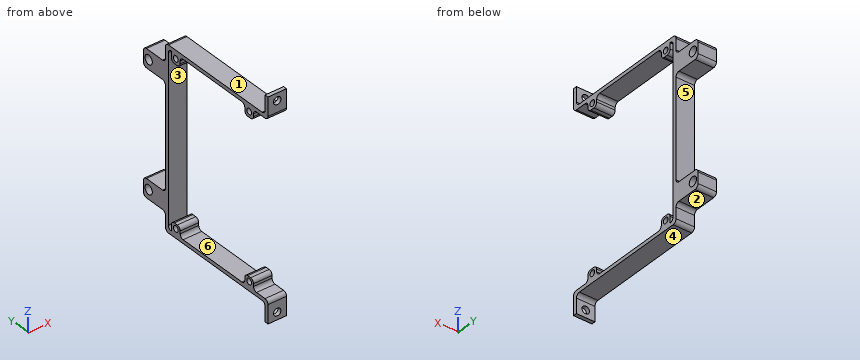
```python
from build123d import *

# Parameters (mm, degrees)
SKETCH1_W             = 10
SKETCH1_H             = 15
SKETCH1_R             = 2.5
BOSS_EXTRUDE1_DEPTH   = 10
FILLET1_R             = 2
F_4_0MM_DOWEL_HOLE1_D = 4
SKETCH4_W             = 5.416503596
SKETCH4_H             = 6
SKETCH4_R             = 1.6
BOSS_EXTRUDE2_DEPTH   = 10
FILLET1_OF_MIRROR1_R  = 2
SKETCH5_W             = 5.416503596
SKETCH5_H             = 6
SKETCH5_R             = 1.6
BOSS_EXTRUDE3_DEPTH   = 10
FILLET2_R             = 2


with BuildPart() as part:
    # Sketch1 → Boss-Extrude1 (new body)
    # profile 1 of 2: a face of its own
    with BuildSketch(Plane(origin=(0, 0, 0), x_dir=(0, 0, -1), z_dir=(1, 0, 0))):
        with Locations((-33.5, 77.5)):
            Rectangle(SKETCH1_W, SKETCH1_H)
        with Locations((-33.5, 81.5)):
            Circle(SKETCH1_R, mode=Mode.SUBTRACT)
    # profile 2 of 2: a face of its own
    with BuildSketch(Plane(origin=(0, 0, 0), x_dir=(0, 0, -1), z_dir=(1, 0, 0))):
        Polygon((-46.5, 68), (0, 68), (0, 70), (-48.5, 70), (-48.5, 2), (-58.5, 2), (-58.5, 0), (-46.5, 0), align=None)
    boss_extrude1 = extrude(amount=BOSS_EXTRUDE1_DEPTH)

    # Fillet1
    fillet1_edges = [part.edges().sort_by_distance(p)[0] for p in [
        (5, 68, 46.5),
        (5, 2, 48.5),
        (5, 70, 48.5),
    ]]
    fillet(fillet1_edges, radius=FILLET1_R)

    # Ø4.0mm Dowel Hole1 (through all)
    with Locations(Plane(origin=(5, 2, 54.5), x_dir=(0, 0, 1), z_dir=(0, 1, 0))):
        with Locations((0, 0)):
            f_4_0mm_dowel_hole1 = Hole(F_4_0MM_DOWEL_HOLE1_D / 2)

    # Sketch4 → Boss-Extrude2 (add)
    # profile 1 of 2: a face of its own
    with BuildSketch(Plane(origin=(10, 0, 0), x_dir=(0, 0, -1), z_dir=(1, 0, 0))):
        with Locations((-43.791748202, 62.946385234)):
            Rectangle(SKETCH4_W, SKETCH4_H)
        with Locations((-44.083496404, 62.946385234)):
            Circle(SKETCH4_R, mode=Mode.SUBTRACT)
    # profile 2 of 2: a face of its own
    with BuildSketch(Plane(origin=(10, 0, 0), x_dir=(0, 0, -1), z_dir=(1, 0, 0))):
        with Locations((-43.791748202, 12.852385234)):
            Rectangle(SKETCH4_W, SKETCH4_H)
        with Locations((-44.083496404, 12.852385234)):
            Circle(SKETCH4_R, mode=Mode.SUBTRACT)
    extrude(amount=-BOSS_EXTRUDE2_DEPTH)

    # Mirror1: Boss-Extrude1, Ø4.0mm Dowel Hole1 across plane
    add(boss_extrude1.mirror(Plane.XY))
    add(f_4_0mm_dowel_hole1.mirror(Plane.XY), mode=Mode.SUBTRACT)

    # Fillet1 of Mirror1
    fillet1_of_mirror1_edges = [part.edges().sort_by_distance(p)[0] for p in [
        (5, 68, -46.5),
        (5, 2, -48.5),
        (5, 70, -48.5),
    ]]
    fillet(fillet1_of_mirror1_edges, radius=FILLET1_OF_MIRROR1_R)

    # Sketch5 → Boss-Extrude3 (add)
    # profile 1 of 2: a face of its own
    with BuildSketch(Plane(origin=(10, 0, 0), x_dir=(0, 0, -1), z_dir=(1, 0, 0))):
        with Locations((43.791748202, 62.946385234)):
            Rectangle(SKETCH5_W, SKETCH5_H)
        with Locations((43.602503596, 62.946385234)):
            Circle(SKETCH5_R, mode=Mode.SUBTRACT)
    # profile 2 of 2: a face of its own
    with BuildSketch(Plane(origin=(10, 0, 0), x_dir=(0, 0, -1), z_dir=(1, 0, 0))):
        with Locations((43.791748202, 12.852385234)):
            Rectangle(SKETCH5_W, SKETCH5_H)
        with Locations((43.602503596, 12.852385234)):
            Circle(SKETCH5_R, mode=Mode.SUBTRACT)
    extrude(amount=-BOSS_EXTRUDE3_DEPTH)

    # Fillet2
    fillet2_edges = [part.edges().sort_by_distance(p)[0] for p in [
        (5, 70, -38.5),
        (5, 85, -38.5),
        (5, 85, -28.5),
        (5, 70, -28.5),
        (5, 0, -46.5),
        (5, 65.946385234, -41.083496404),
        (5, 59.946385234, -41.083496404),
        (5, 59.946385234, -46.5),
        (5, 15.852385234, -46.5),
        (5, 15.852385234, -41.083496404),
        (5, 9.852385234, -41.083496404),
        (5, 9.852385234, -46.5),
        (5, 85, 38.5),
        (5, 85, 28.5),
        (5, 70, 28.5),
        (5, 0, 46.5),
        (5, 70, 38.5),
        (5, 65.946385234, 41.083496404),
        (5, 59.946385234, 41.083496404),
        (5, 59.946385234, 46.5),
        (5, 15.852385234, 41.083496404),
        (5, 15.852385234, 46.5),
        (5, 9.852385234, 46.5),
        (5, 9.852385234, 41.083496404),
    ]]
    fillet(fillet2_edges, radius=FILLET2_R)


solid = part.part
```
Model file for the job. Use its own axes, mm. Face numbers are marked on the shaded views. A direction names the side the tool comes from. Coordinates: 2 decimals unless noted, no trailing zeros. Order: outer loops, then holes, each group sorted by start corner. A loop starts at its lowest first (then second) coordinate and runs counter-clockwise, first axis right, second up. Notation, with made-up numbers: (86, -22) -> (98, -22) arc R22 ccw to (98, -6) -> close; hole circle Ø2 at (-3, -38.75). An arc over 180 degrees is marked (long way). Answer as a JSON object with one key per item and string values. Group by question number.
1) Cut at B-B, the plane y = 81.5. Write the cut outline in (x, z).
2) Flat gauge pins, fed straight in: pin 1 (1.5 mm diameter, centred on x = 7, y = 52.5, fed in from -Z); pin 2 (2 mm diameter, centred on x = 5, z = 38, fed in from -Y); pin 3 (3 mm diameter, centred on x = 6.5, z = -44.5, fed in from +Y); pin 4 (4.5 mm diameter, centred on x = 6.5, y = 4, fed in from +Z). Where does each tip first touch, or does it go through?
3) Cut at A-A, the plane z = -54.5. Write the cut outline in (x, y).
4) Drill centre lines: L1, parallel to Z at x = 6.25, y = 34; L2, parallel to Y at x = 3.5, z = 33.5; L3, parallel to Z at x = 1, y = 12. Where is each one in solid material? Low to high.
5) Cut at D-D, the plane x = 5. Count the separate pieces of the cut face and the enclosed holes in it, then the cut area to 3 significant figures.
6) Cut at C-C, the plane y = 28. Write the cut outline in (x, z).
7) Which spindle directions (+Z, -Z, +X, -X, +Y, -Y) get a long thin tool onto all of the face, cutting with end or side? Do the marked faces 4, 5 and 6. Say none if no direction does.
8) Pull direction Z, two halves, no side cores. Call the marked faces 1, 2 and 3: +Z half, -Z half, draft (parallel to the pull), parting line (faces both ways), or undercut.
Check values:
{
 "1": {"outline": "(0, -38.5) -> (10, -38.5) -> (10, -36) -> (0, -36) -> close; (0, -31) -> (10, -31) -> (10, -28.5) -> (0, -28.5) -> close; (0, 28.5) -> (10, 28.5) -> (10, 31) -> (0, 31) -> close; (0, 36) -> (10, 36) -> (10, 38.5) -> (0, 38.5) -> close"},
 "2": {"pin 1": "stops at z = -48.5", "pin 2": "stops at y = 68", "pin 3": "stops at y = 70", "pin 4": "stops at z = 58.5"},
 "3": {"outline": "(0, 0) -> (3, 0) -> (3, 2) -> (0, 2) -> close; (7, 0) -> (10, 0) -> (10, 2) -> (7, 2) -> close"},
 "4": {"L1": "z = -48.5 to -46.5, 46.5 to 48.5", "L2": "y = 68 to 79, 84 to 85", "L3": "z = -48.5 to -44.96, -42.25 to -41.08, 41.08 to 42.73, 45.44 to 48.5"},
 "5": {"separate pieces": "3", "enclosed holes": "6", "area": "847 mm²"},
 "6": {"outline": "(0, -48.5) -> (10, -48.5) -> (10, -46.5) -> (0, -46.5) -> close; (0, 46.5) -> (10, 46.5) -> (10, 48.5) -> (0, 48.5) -> close"},
 "7": {"face 4": "-Z, +X, -X, +Y", "face 5": "+X, -X, +Y", "face 6": "+X, -X"},
 "8": {"face 1": "+Z half", "face 2": "-Z half", "face 3": "undercut"}
}
